Geometry check sheet. Reference: the model listing, model coordinates, mm. Coordinates: 2 decimals unless noted, no trailing zeros. Write each loop counter-clockwise with the first axis right and the second up, starting at its lowest first coordinate (ties: lowest second). Pieces come first, ordered by that corner, then holes. Notation, with made-up numbers: (64.25, 70) -> (101.25, 70) arc R16 ccw to (101.25, 99) -> close; hole circle Ø8 at (25.5, -20.75). An arc over 180 degrees is marked (long way). Answer in a Markdown table with one row per item. Add a question column.
1. Cross-section at A-A on x = 42. Record the cut outline in (y, z), and give its area (3 significant figures).
2. Scan lines: L1, parallel to Y at x = 45.75, z = 4; L2, parallel to Z at x = 40.5, y = 6; L3, parallel to Y at x = 42, z = 6.75. Record each from-to range of solid material in increasing order. Write a range as from..to.
3. Cross-section at B-B on y = 0. Record the cut outline in (x, z).
```python
from build123d import *

# Parameters (mm, degrees)
SKETCH_1_W                      = 94
SKETCH_1_H                      = 20
EXTRUDE_1_DEPTH                 = 8
M4_ALTADJUST_D                  = 3.3
M4_ALTADJUST_DEPTH              = 8
M3_HORIZONTALBAR_FIX_AT_2_COUNT = 2
M3_HORIZONTALBAR_FIX_AT_2_PITCH = 12


with BuildPart() as part:
    # 스케치1 → 보스-돌출1 (new body)
    with BuildSketch(Plane.XY):
        Rectangle(SKETCH_1_W, SKETCH_1_H)
    extrude(amount=EXTRUDE_1_DEPTH)

    # M4-ALTADJUST
    with Locations(Plane.XY.offset(8)):
        with Locations((42, 0)):
            Hole(M4_ALTADJUST_D / 2, depth=M4_ALTADJUST_DEPTH)

    # 스케치5 → M3-HORIZONTALBAR_FIX (revolve, cut)
    with BuildSketch(Plane(origin=(47, 6, 4), x_dir=(0, 0, -1), z_dir=(0, 1, 0))):
        Polygon((0, 0), (0, 9.251075774), (1.25, 8.5), (1.25, 0), align=None)
    m3_horizontalbar_fix = revolve(axis=Axis((53.35, 6, 4), (-1, 0, 0)), mode=Mode.SUBTRACT)

    # M3-HORIZONTALBAR_FIX at 2: M3-HORIZONTALBAR_FIX ×2
    with Locations(*[(0, -i * M3_HORIZONTALBAR_FIX_AT_2_PITCH, 0) for i in range(1, M3_HORIZONTALBAR_FIX_AT_2_COUNT)]):
        add(m3_horizontalbar_fix, mode=Mode.SUBTRACT)

    # 대칭 복사1: M3-HORIZONTALBAR_FIX across plane
    add(m3_horizontalbar_fix.mirror(Plane(origin=(0, 0, 0), x_dir=(0, 0, 1), z_dir=(1, 0, 0))), mode=Mode.SUBTRACT)

    # 대칭 복사1 copy 1 sketch → 대칭 복사1 copy 1 (revolve, cut)
    with BuildSketch(Plane(origin=(-47, -6, 4), x_dir=(0, 0, -1), z_dir=(0, 1, 0))):
        Polygon((0, 0), (0, -9.251075774), (1.25, -8.5), (1.25, 0), align=None)
    revolve(axis=Axis((-53.35, -6, 4), (-1, 0, 0)), mode=Mode.SUBTRACT)


solid = part.part
```
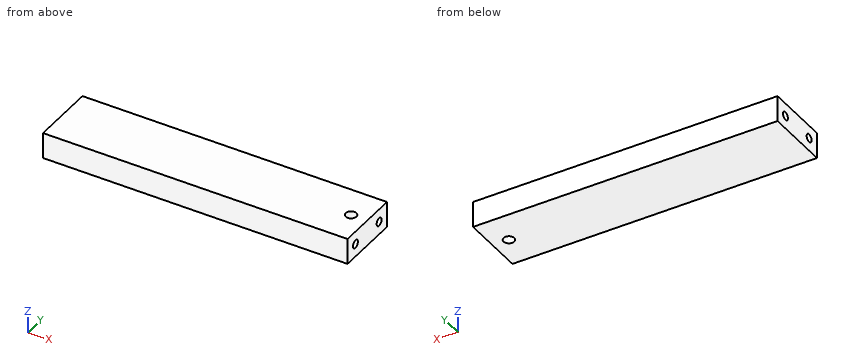
Results found:
| question | item | result |
|---|---|---|
| 1 | outline | (-10, 0) -> (-1.65, 0) -> (-1.65, 8) -> (-10, 8) -> close; (1.65, 0) -> (10, 0) -> (10, 8) -> (1.65, 8) -> close; hole circle Ø2.5 at (-6, 4); hole circle Ø2.5 at (6, 4) |
| 1 | area | 124 mm^2 |
| 2 | L1 | y = -10..-7.25, -4.75..4.75, 7.25..10 |
| 2 | L2 | z = 0..2.75, 5.25..8 |
| 2 | L3 | y = -10..-1.65, 1.65..10 |
| 3 | outline | (-47, 0) -> (40.35, 0) -> (40.35, 8) -> (-47, 8) -> close; (43.65, 0) -> (47, 0) -> (47, 8) -> (43.65, 8) -> close |
